Design review of the part built by this model. Coordinates are the model's own, in mm. Face numbers are marked on the shaded views. A direction names the side the tool comes from. Round coordinates to 2 decimals unless told otherwise and drop trailing zeros. Loops run counter-clockwise (first coordinate to the right, second up) from the corner with the lowest first, then second, coordinate; pieces in that order, holes last. Notation, with made-up numbers: (-31, -27) - (-6, -27) arc R21 ccw to (-6, -8) - close; hole circle Ø4 at (21.5, 74.25). An arc over 180 degrees is marked (long way). Use one line per item in the form item = value. Start each with the question number.
(1) Wall thickness on probe 1 along Z at (x, y) = (0, -20.8); probe 2 along X at (y, z) = (21.5, 150.5); probe 3 along Z at (x, y) = (0, -23.05): over which ranges is each line inside the solid? List them lowest first. Write a range as [from, to].
(2) We need section A-A, the plane x = 0. Write out the cut boundary in (y, z), then the cut area to 4 significant figures.
(3) We need section D-D, the plane y = 12. Write out the cut boundary in (x, z).
(4) Machinability: for the marked faces 4 and 5, which of the approach directions +Z, -Z, +X, -X, +Y, -Y give a long, thin tool a straight path to every point of the face, cutting with its end or side? Answer none if there is none.
(5) The part is to be moulded in two halves that separate along X. For the marked faces 1, 2 and 3, say which applies: released by +X, released by -X, zero draft, split by the parting line, or undercut.
(6) We need section C-C, the plane z = 97.5. Write out the cut boundary in (x, y).
(7) For pin 1 (1.5 mm diameter, centred on x = -76, z = 44, fed in from +Y); pin 2 (10 mm diameter, centred on y = 26.5, z = 39.5, fed in from +X); pin 3 (15 mm diameter, centred on x = 6.5, z = 75, fed in from -Y), all flat-tipped, find the tip position at first contact; note any pin that passes through.
(8) We need section B-B, the plane y = 1.5. Write out the cut boundary in (x, z).
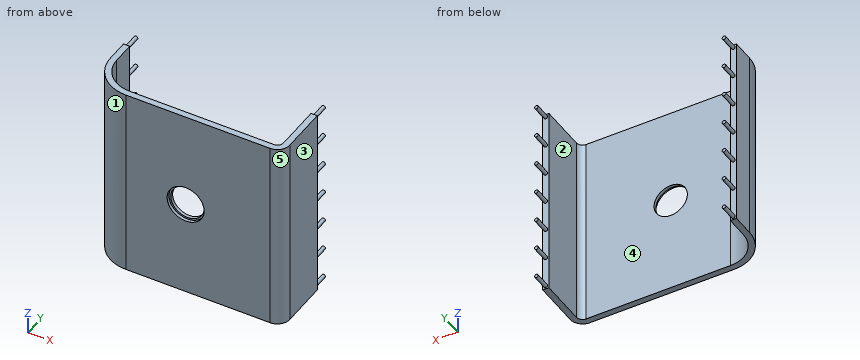
from build123d import *

# Parameters (mm, degrees)
F1_DEPTH = 157
F2_R     = 13.5
F3_DEPTH = 25
F4_R     = 15
F5_DEPTH = 2.5
F6_R     = 1.475
F7_DEPTH = 13
F8_R     = 1.475
F9_DEPTH = 13


with BuildPart() as f1:
    # F0 (on Top) → F1 (new body)
    with BuildSketch(Plane.XY):
        with BuildLine():
            Line((-48.5, -24), (68.5, -24))
            ThreePointArc((68.5, -24), (75.571068, -21.071068), (78.5, -14))
            Line((78.5, -14), (78.5, 24))
            Line((78.5, 24), (73.5, 24))
            Line((73.5, 24), (73.5, -14))
            ThreePointArc((73.5, -14), (72.035534, -17.535534), (68.5, -19))
            Line((68.5, -19), (-48.499, -19))
            ThreePointArc((-48.499, -19), (-66.177377, -11.677377), (-73.5, 6.001))
            Line((-73.5, 6.001), (-73.5, 24))
            Line((-73.5, 24), (-78.5, 24))
            Line((-78.5, 24), (-78.5, 6))
            ThreePointArc((-78.5, 6), (-69.713203, -15.213203), (-48.5, -24))
        make_face()
    extrude(amount=F1_DEPTH)

    # F2 (on face) → F3 (cut)
    with BuildSketch(Plane.XZ.offset(24)):
        with Locations((0, 78.5)):
            Circle(F2_R)
    extrude(amount=-F3_DEPTH, mode=Mode.SUBTRACT)

    # F4 (on face) → F5 (cut)
    with BuildSketch(Plane.XZ.offset(24)):
        with Locations((0, 78.5)):
            Circle(F4_R)
    extrude(amount=-F5_DEPTH, mode=Mode.SUBTRACT)

    # F6 (on face) → F7 (join)
    with BuildSketch(Plane(origin=(0, 24, 0), x_dir=(-1, 0, 0), z_dir=(0, 1, 0))):
        with Locations((-76, 154.5)):
            Circle(F6_R)
        with Locations((-76, 129.1667)):
            Circle(F6_R)
        with Locations((-76, 103.8334)):
            Circle(F6_R)
        with Locations((-76, 78.5001)):
            Circle(F6_R)
        with Locations((-76, 53.1668)):
            Circle(F6_R)
        with Locations((-76, 27.8335)):
            Circle(F6_R)
        with Locations((-76, 2.5002)):
            Circle(F6_R)
    extrude(amount=F7_DEPTH)

    # F8 (on face) → F9 (join)
    with BuildSketch(Plane(origin=(0, 24, 0), x_dir=(-1, 0, 0), z_dir=(0, 1, 0))):
        with Locations((76, 103.8334)):
            Circle(F8_R)
        with Locations((76, 129.1667)):
            Circle(F8_R)
        with Locations((76, 154.5)):
            Circle(F8_R)
        with Locations((76, 78.5001)):
            Circle(F8_R)
        with Locations((76, 53.1668)):
            Circle(F8_R)
        with Locations((76, 2.5002)):
            Circle(F8_R)
        with Locations((76, 27.8335)):
            Circle(F8_R)
    extrude(amount=F9_DEPTH)


solid = f1.part
Data:
q1.probe_1 = [0, 65], [92, 157]
q1.probe_2 = [-78.5, -73.5], [73.5, 78.5]
q1.probe_3 = [0, 63.5], [93.5, 157]
q2.outline = (-24, 0) - (-19, 0) - (-19, 65) - (-21.5, 65) - (-21.5, 63.5) - (-24, 63.5) - close; (-24, 93.5) - (-21.5, 93.5) - (-21.5, 92) - (-19, 92) - (-19, 157) - (-24, 157) - close
q2.area = 642.5 mm^2
q3.outline = (-78.5, 0) - (-73.5, 0) - (-73.5, 157) - (-78.5, 157) - close; (73.5, 0) - (78.5, 0) - (78.5, 157) - (73.5, 157) - close
q4.face_4 = +Z, -Z, +Y
q4.face_5 = +Z, -Z, +X, -Y
q5.face_1 = released by -X
q5.face_2 = undercut
q5.face_3 = released by +X
q6.outline = (-78.5, 6) arc R30 ccw to (-48.5, -24) - (68.5, -24) arc R10 ccw to (78.5, -14) - (78.5, 24) - (73.5, 24) - (73.5, -14) arc R5 cw to (68.5, -19) - (-48.5, -19) arc R25 cw to (-73.5, 6) - (-73.5, 24) - (-78.5, 24) - close
q7.pin_1 = 24
q7.pin_2 = 78.5
q7.pin_3 = -21.5
q8.outline = (-78.16, 0) - (-73.09, 0) - (-73.09, 157) - (-78.16, 157) - close; (73.5, 0) - (78.5, 0) - (78.5, 157) - (73.5, 157) - close
